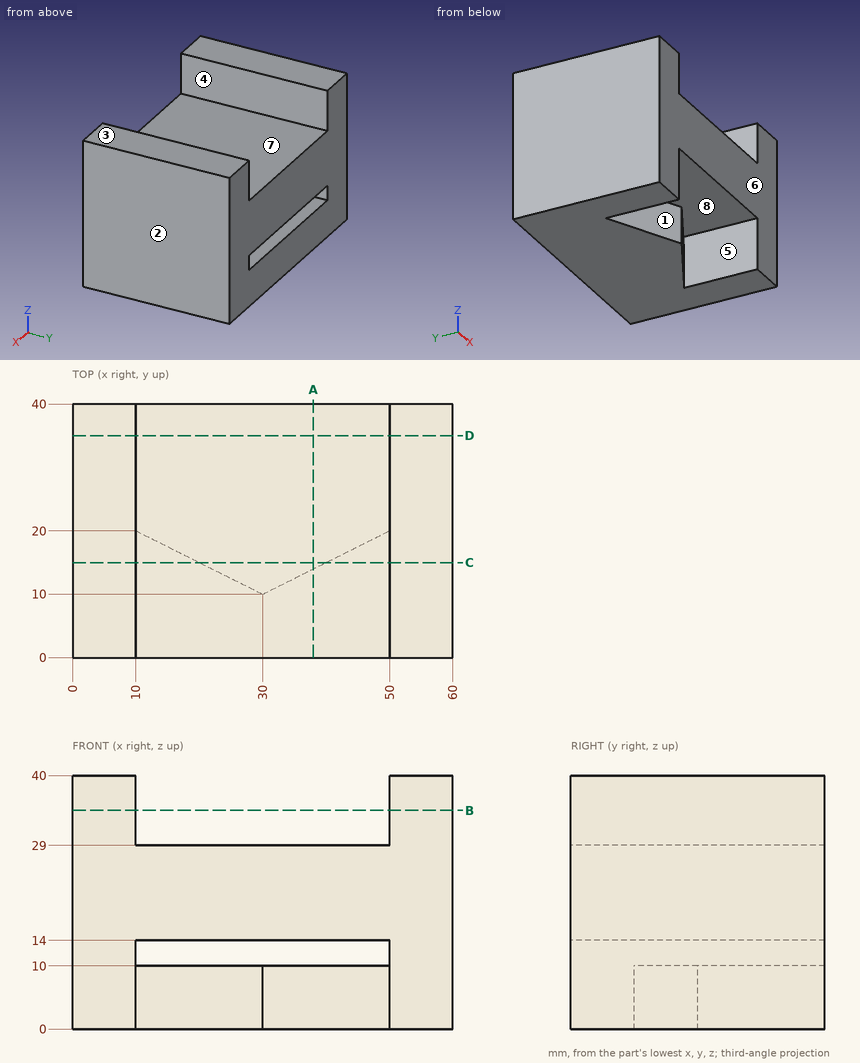
Geometry: see drawing. Coordinates: mm, zero at the bounding-box minimum. A direction names the side the tool comes from. Round coordinates to 2 decimals unless told otherwise and drop trailing zeros. Write each loop counter-clockwise with the first axis right and the second up, starting at its lowest first coordinate (ties: lowest second). Pieces come first, ordered by that corner, then holes. Notation, with made-up numbers: (-7.75, -4) - (7.25, -4) arc R20 ccw to (7.25, 8) - close; hole circle Ø10 at (-19, -39). An arc over 180 degrees is marked (long way). Use CSV: the item, a comma, the result in double quotes. Start each with the question number.
(1) Set-up query: the marked faces 5, 6, 7 and 8. Return all of +Z, -Z, +X, -X, +Y, -Y with unobstructed straight access to the full face (end or side cutting, diameter ignored); none if empty.
(2) Material intervals for probe 1 along Z at (x, y) = (16.5, 31); probe 2 along X at (y, z) = (2, 3.5); probe 3 along Z at (x, y) = (27.5, 9.5), sorted ascending. Write a range as [from, to].
(3) Cut plane B-B, the plane z = 34.5. Return loops of the section in (x, y).
(4) Mould query, pull axis X, two halves, no side actions, for the marked faces 1, 2, 3 and 4. Classes: pulls with the +X half, pulls with the -X half, needs draft (parallel to the pull), parting line crosses it, or undercut.
(5) Cut plane C-C, the plane y = 15. Return loops of the section in (x, z).
(6) Cut plane A-A, the plane x = 38. Return loops of the section in (y, z).
(7) First-contact query: pin 1 Ø2 at (x, y) = (20.5, 9.5) entering from -Z; pin 2 Ø12 at (x, y) = (21.5, 21.5) entering from +Z. Flat tips, straight axial feed; report the tip coordinate or a pass-through.
(8) Cut plane D-D, the plane y = 35. Return loops of the section in (x, z), and give its area (3 significant figures).
Geometry says:
1,face 5,"-Y"
1,face 6,"+Z, -Z, +X, -X, -Y"
1,face 7,"+Z, +Y, -Y"
1,face 8,"+Y, -Y"
2,probe 1,"[0, 10], [14, 29]"
2,probe 2,"[0, 10], [50, 60]"
2,probe 3,"[14, 29]"
3,outline,"(0, 0) - (10, 0) - (10, 40) - (0, 40) - close; (50, 0) - (60, 0) - (60, 40) - (50, 40) - close"
4,face 1,"undercut"
4,face 2,"pulls with the +X half"
4,face 3,"needs draft"
4,face 4,"undercut"
5,outline,"(0, 0) - (10, 0) - (10, 14) - (50, 14) - (50, 0) - (60, 0) - (60, 40) - (50, 40) - (50, 29) - (10, 29) - (10, 40) - (0, 40) - close; (20, 0) - (40, 0) - (40, 10) - (20, 10) - close"
6,outline,"(0, 14) - (40, 14) - (40, 29) - (0, 29) - close; (14, 0) - (40, 0) - (40, 10) - (14, 10) - close"
7,pin 1,"z = 14"
7,pin 2,"z = 29"
8,outline,"(0, 0) - (60, 0) - (60, 40) - (50, 40) - (50, 29) - (10, 29) - (10, 40) - (0, 40) - close; hole (10, 10) - (50, 10) - (50, 14) - (10, 14) - close"
8,area,"1,800 mm²"
